```python
from build123d import *

# Parameters (mm, degrees)
BOSS_EXTRUDE1_DEPTH = 18
FILLET1_R           = 40


with BuildPart() as part:
    # Sketch1 → Boss-Extrude1 (new body)
    with BuildSketch(Plane.XY):
        with BuildLine():
            Line((-27, 0), (27, 0))
            add(Edge.make_bspline(
                [(27, 0), (27, -49.026425591), (64.594351551, -134.908704781), (110, -200)],
                knots=[0, 0, 0, 0, 1, 1, 1, 1], degree=3))
            Line((110, -200), (-110, -200))
            add(Edge.make_bspline(
                [(-27, 0), (-27, -49.026425591), (-64.594351551, -134.908704781), (-110, -200)],
                knots=[0, 0, 0, 0, 1, 1, 1, 1], degree=3))
        make_face()
    extrude(amount=BOSS_EXTRUDE1_DEPTH)

    # Fillet1
    fillet1_edges = [part.edges().sort_by_distance(p)[0] for p in [
        (-110, -200, 9),
        (110, -200, 9),
    ]]
    fillet(fillet1_edges, radius=FILLET1_R)


solid = part.part
```
Work out the finished part from the listing and answer in its coordinate system (mm). Give positions to 0.01 mm unless a question says otherwise; leave off trailing zeros. Return JSON: item names as keys, results as strings.
1) For a pull along Y with two mould halves and no side action, classify faces 1 (the flat face through (0, 0, 9)), 2 (the flat face through (1, -200, 9)), 3 (the flat face through (1, -121, 0)) as +Y half, -Y half, draft (parallel to the pull), parting line (faces both ways), or undercut.
Resolved:
{"face 1": "+Y half", "face 2": "-Y half", "face 3": "draft"}
2) Straight lines are drawn through the part: line 1 along X through (y, z) = (-159.5, 5.75); line 2 along Y through (x, z) = (-67, 11.75); line 3 along X through (y, z) = (-127, 4). For each, find the intervals that lie inside material, in ascending order. Write a range as [from, to].
Resolved:
{"line 1": "[-78.77, 78.77]", "line 2": "[-188.35, -127.54]", "line 3": "[-66.73, 66.73]"}
3) Each of these flat-tipped pins is pushed along its axis until it touches: pin 1 (6 mm diameter, centred on y = -102.5, z = 6.5, fed in from +X); pin 2 (6 mm diameter, centred on x = 11.5, z = 12, fed in from +Y); pin 3 (6 mm diameter, centred on y = -89, z = 2.5, fed in from +X); pin 4 (8 mm diameter, centred on x = 50.5, z = 14.5, fed in from -Y). Where does it stop, or does it pass through?
Resolved:
{"pin 1": "x = 56.5", "pin 2": "y = 0", "pin 3": "x = 50.64", "pin 4": "y = -199.25"}
